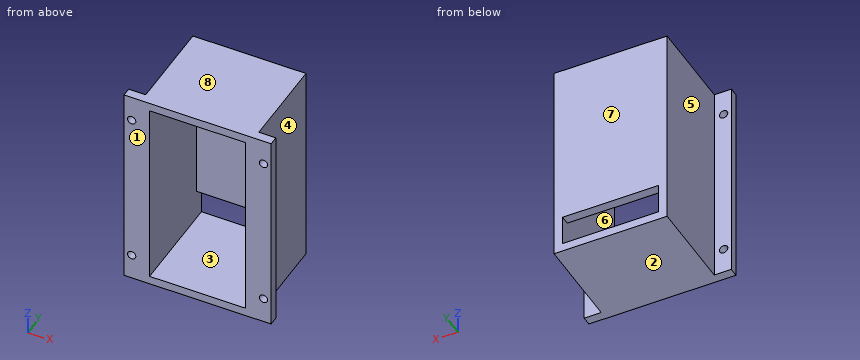
```python
from build123d import *

# Parameters (mm, degrees)
SKETCH2_W           = 37.1
SKETCH2_H           = 68.6
BOSS_EXTRUDE1_DEPTH = 33
SKETCH1_W           = 31.5
SKETCH1_H           = 63
CUT_EXTRUDE1_DEPTH  = 30
SKETCH3_W           = 31.5
SKETCH3_H           = 10
CUT_EXTRUDE2_DEPTH  = 5
SKETCH6_W           = 5.575
SKETCH6_H           = 68.6
SKETCH6_R           = 1.375
BOSS_EXTRUDE2_DEPTH = 3


with BuildPart() as part:
    # Sketch2 → Boss-Extrude1 (new body)
    with BuildSketch(Plane(origin=(0, 0, 0), x_dir=(1, 0, 0), z_dir=(0, 1, 0))):
        with Locations((15.75, 31.5)):
            Rectangle(SKETCH2_W, SKETCH2_H)
    extrude(amount=BOSS_EXTRUDE1_DEPTH)

    # Sketch1 → Cut-Extrude1 (cut)
    with BuildSketch(Plane(origin=(0, 0, 0), x_dir=(1, 0, 0), z_dir=(0, 1, 0))):
        with Locations((15.75, 31.5)):
            Rectangle(SKETCH1_W, SKETCH1_H)
    extrude(amount=CUT_EXTRUDE1_DEPTH, mode=Mode.SUBTRACT)

    # Sketch3 → Cut-Extrude2 (cut)
    with BuildSketch(Plane.XZ.offset(-30)):
        with Locations((15.75, -58)):
            Rectangle(SKETCH3_W, SKETCH3_H)
    extrude(amount=-CUT_EXTRUDE2_DEPTH, mode=Mode.SUBTRACT)

    # Sketch6 → Boss-Extrude2 (add)
    # profile 1 of 2: a face of its own
    with BuildSketch(Plane.XZ):
        with Locations((37.0875, -31.5)):
            Rectangle(SKETCH6_W, SKETCH6_H)
        with Locations(Location((37.375, -57.175, 0), (0, 0, 270))):
            Circle(SKETCH6_R, mode=Mode.SUBTRACT)
        with Locations(Location((37.375, -5.825, 0), (0, 0, 90))):
            Circle(SKETCH6_R, mode=Mode.SUBTRACT)
    # profile 2 of 2: a face of its own
    with BuildSketch(Plane.XZ):
        with Locations((-5.5875, -31.5)):
            Rectangle(SKETCH6_W, SKETCH6_H)
        with Locations(Location((-5.875, -5.825, 0), (0, 0, 270))):
            Circle(SKETCH6_R, mode=Mode.SUBTRACT)
        with Locations(Location((-5.875, -57.175, 0), (0, 0, 90))):
            Circle(SKETCH6_R, mode=Mode.SUBTRACT)
    extrude(amount=-BOSS_EXTRUDE2_DEPTH)


solid = part.part
```
Read the model definition and answer for the solid it produces. Units are mm, in the model's axes. Face numbers are marked on the shaded views. A direction names the side the tool comes from. Coordinates: 2 decimals unless noted, no trailing zeros. Order: outer loops, then holes, each group sorted by start corner. A loop starts at its lowest first (then second) coordinate and runs counter-clockwise, first axis right, second up. Notation, with made-up numbers: (-26, -10) - (-13, -10) arc R17 cw to (-13, 15) - close; hole circle Ø1 at (78.5, -31). An arc over 180 degrees is marked (long way). Answer as a JSON object with one key per item and string values. Group by question number.
Item 1: Consider probe 1 along Z at (x, y) = (4.5, 20); probe 2 along X at (y, z) = (7, -24); probe 3 along X at (y, z) = (2, -14.5) (3 decimals). Determine where each line is inside the solid, lowest interval first. Write a range as from..to.
Item 2: The mould has two halves that part along Z. Classify the marked faces 1, 2 and 3: +Z half, -Z half, draft (parallel to the pull), parting line (faces both ways), or undercut.
Item 3: Section B-B (y = 12) is taken. Give the vertices of the cut face in (x, z).
Item 4: A tool of negligible diameter and unlimited length cuts with its end or side. For the marked faces 4, 5, 6, 7 and 8, from which of +Z, -Z, +X, -X, +Y, -Y can it reach the whole face along a straight path? Write none if from no direction.
Item 5: Section A-A (x = 28.5) is taken. Give the vertices of the cut face in (y, z), plus the area to 3 significant figures.
Item 6: Section D-D (y = 2) is taken. Give the vertices of the cut face in (x, z) (3 decimals), plus the area to 3 significant figures.
Item 7: Section C-C (z = -35) is taken. Give the vertices of the cut face in (x, y) (3 decimals), plus the area to 3 significant figures.
Item 8: Flat-ended cylindrical pins translate along their axes: P1, Ø3, axis at x = 36, z = -25.5, coming from the +Y side; P2, Ø12, axis at y = 20, z = -45.5, coming from the +X side; P3, Ø9, axis at y = 22, z = -27.5, coming from the -X side; P4, Ø2.5, axis at x = 37.375, z = -57.175, coming from the -Y side. Find the tip coordinate at first contact, or state that the pin passes through.
Results are:
{
 "1": {"probe 1": "z = -65.8..-63, 0..2.8", "probe 2": "x = -2.8..0, 31.5..34.3", "probe 3": "x = -8.375..0, 31.5..39.875"},
 "2": {"face 1": "draft", "face 2": "-Z half", "face 3": "undercut"},
 "3": {"outline": "(-2.8, -65.8) - (34.3, -65.8) - (34.3, 2.8) - (-2.8, 2.8) - close; hole (0, -63) - (31.5, -63) - (31.5, 0) - (0, 0) - close"},
 "4": {"face 4": "+Z, -Z, +X, +Y", "face 5": "+Z, -Z, -X, +Y", "face 6": "-Y", "face 7": "+Z, -Z, +X, -X, +Y", "face 8": "+Z, +X, -X, +Y, -Y"},
 "5": {"outline": "(0, -65.8) - (33, -65.8) - (33, -63) - (0, -63) - close; (0, 0) - (30, 0) - (30, -53) - (33, -53) - (33, 2.8) - (0, 2.8) - close", "area": "344 mm^2"},
 "6": {"outline": "(-8.375, -65.8) - (39.875, -65.8) - (39.875, 2.8) - (-8.375, 2.8) - close; hole circle Ø2.75 at (-5.875, -57.175); hole circle Ø2.75 at (-5.875, -5.825); hole (0, -63) - (31.5, -63) - (31.5, 0) - (0, 0) - close; hole circle Ø2.75 at (37.375, -57.175); hole circle Ø2.75 at (37.375, -5.825)", "area": "1,300 mm^2"},
 "7": {"outline": "(-8.375, 0) - (0, 0) - (0, 30) - (31.5, 30) - (31.5, 0) - (39.875, 0) - (39.875, 3) - (34.3, 3) - (34.3, 33) - (-2.8, 33) - (-2.8, 3) - (-8.375, 3) - close", "area": "313 mm^2"},
 "8": {"P1": "stops at y = 3", "P2": "stops at x = 34.3", "P3": "stops at x = -2.8", "P4": "passes through"}
}
